Could you check a few things on this model? Use its own coordinates, in mm. Face numbers are marked on the shaded views. A direction names the side the tool comes from. Give positions to 0.01 mm unless a question says otherwise; leave off trailing zeros. Loops run counter-clockwise (first coordinate to the right, second up) from the corner with the lowest first, then second, coordinate; pieces in that order, holes last. Notation, with made-up numbers: M 63.25,17 L 113.25,17 A22 ccw 113.25,47 Z; hole C 77.25,5.25 d1. An arc over 180 degrees is marked long. Return JSON: item names as keys, results as strings. Group by question number.
1. Please list where these lines run through material, in increasing order: line 1 (X direction, y = 3, z = 32); line 2 (Z direction, x = 47, y = 16); line 3 (X direction, y = 8, z = 11.5).
2. If we mould it in two halves opening along Y, with no side actions, what happens to the marked faces 4, 5, 6 and 7? For each: +Y half, -Y half, draft (parallel to the pull), parting line (faces both ways), or undercut.
3. For the marked faces 1, 2 and 3, which set-ups out of +Z, -Z, +X, -X, +Y, -Y let a thin tool reach every point of the face, with its end or its side?
4. If we section it at B-B (x = 52.5): Write out the boundary of the cut face in (y, z), plus the area to 3 significant figures.
5. If we section it at D-D (z = 40): Write out the boundary of the cut face in (x, y), plus the area to 3 significant figures.
6. If we section it at A-A (z = 11): Write out the boundary of the cut face in (x, y).
7. If we section it at C-C (y = 29.5): Write out the boundary of the cut face in (x, z), plus the area to 3 significant figures.
8. For pin 1 (10 mm diameter, centred on y = 24.5, z = 22.5, fed in from -X); pin 2 (15.5 mm diameter, centred on y = 16.5, z = 14, fed in from -X); pin 3 (0.7 mm diameter, centred on x = 30, z = 7.5, fed in from -Y), each with a flat end and sliding along its axis, tell me the tip position at first contact or that it passes through.
```python
from build123d import *

# Parameters (mm, degrees)
F0_W      = 58
F0_H      = 33
F1_DEPTH  = 2
F2_R      = 10
F3_DEPTH  = 15
F4_R      = 4.7
F5_DEPTH  = 14
F6_W      = 12
F6_H      = 1.5
F7_DEPTH  = 34.5
F8_W      = 1.2
F8_H      = 33
F9_DEPTH  = 45
F10_R     = 4.75
F11_DEPTH = 20
F12_W     = 1.2
F12_H     = 33
F13_DEPTH = 45
F14_R     = 9.6
F15_DEPTH = 10
F17_DEPTH = 1.2
F19_DEPTH = 1.2
F20_W     = 9
F20_H     = 45
F21_DEPTH = 1.2
F22_W     = 9
F22_H     = 45
F23_DEPTH = 1.2
F24_SIZE  = 5


with BuildPart() as f1:
    # F0 (on Top) → F1 (new body)
    with BuildSketch(Plane.XY):
        with Locations((29, 16.5)):
            Rectangle(F0_W, F0_H)
    extrude(amount=F1_DEPTH)

    # F2 (on face) → F3 (join)
    with BuildSketch(Plane.XY.offset(2)):
        with Locations((29, 16.5)):
            Circle(F2_R)
    extrude(amount=F3_DEPTH)

    # F4 (on face) → F5 (cut)
    with BuildSketch(Plane.XY.offset(17)):
        with Locations((29, 16.5)):
            Circle(F4_R)
    extrude(amount=-F5_DEPTH, mode=Mode.SUBTRACT)

    # F6 (on Right) → F7 (cut)
    with BuildSketch(Plane.YZ):
        with Locations((15.833333, 7.95)):
            Rectangle(F6_W, F6_H)
    extrude(amount=F7_DEPTH, mode=Mode.SUBTRACT)

    # F8 (on face) → F9 (join)
    with BuildSketch(Plane.XY.offset(2)):
        with Locations((57.4, 16.5)):
            Rectangle(F8_W, F8_H)
    extrude(amount=F9_DEPTH)

    # F10 (on face) → F11 (cut)
    with BuildSketch(Plane.YZ.offset(58)):
        with Locations((16.5, 27)):
            Circle(F10_R)
    extrude(amount=-F11_DEPTH, mode=Mode.SUBTRACT)

    # F12 (on face) → F13 (join)
    with BuildSketch(Plane.XY.offset(2)):
        with Locations((47.2, 16.5)):
            Rectangle(F12_W, F12_H)
    extrude(amount=F13_DEPTH)

    # F14 (on face) → F15 (cut)
    with BuildSketch(Plane.YZ.offset(47.8)):
        with Locations((16.5, 27)):
            Circle(F14_R)
    extrude(amount=-F15_DEPTH, mode=Mode.SUBTRACT)

    # F16 (on Front) → F17 (join)
    with BuildSketch(Plane.XZ):
        Polygon((46.6, 2), (46.6, 47), (29.1, 2), align=None)
    extrude(amount=-F17_DEPTH)

    # F18 (on face) → F19 (join)
    with BuildSketch(Plane(origin=(0, 33, 0), x_dir=(-1, 0, 0), z_dir=(0, 1, 0))):
        Polygon((-29, 2), (-46.6, 47), (-46.6, 2), align=None)
    extrude(amount=-F19_DEPTH)

    # F20 (on Front) → F21 (join)
    with BuildSketch(Plane.XZ):
        with Locations((52.3, 24.5)):
            Rectangle(F20_W, F20_H)
    extrude(amount=-F21_DEPTH)

    # F22 (on face) → F23 (join)
    with BuildSketch(Plane(origin=(0, 33, 0), x_dir=(-1, 0, 0), z_dir=(0, 1, 0))):
        with Locations((-52.3, 24.5)):
            Rectangle(F22_W, F22_H)
    extrude(amount=-F23_DEPTH)

    # F24
    f24_edges = [f1.edges().sort_by_distance(p)[0] for p in [
        (19, 16.5, 17),
    ]]
    chamfer(f24_edges, length=F24_SIZE)


solid = f1.part
```
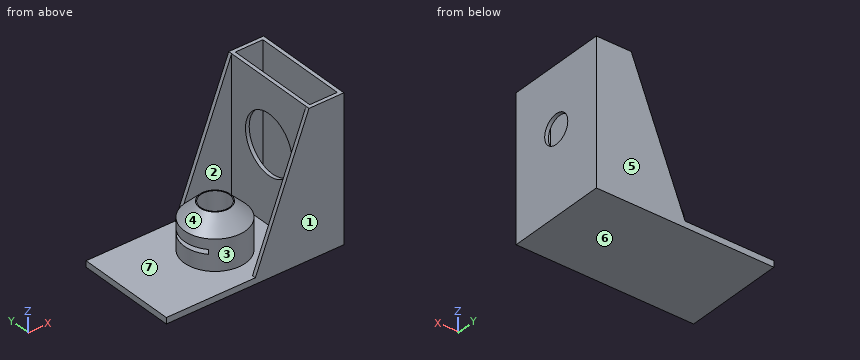
Answer:
{
 "1": {"line 1": "x = 46.6 to 47.8, 56.8 to 58", "line 2": "z = 0 to 17.41, 36.59 to 47", "line 3": "x = 23.73 to 34.27, 46.6 to 47.8, 56.8 to 58"},
 "2": {"face 4": "undercut", "face 5": "+Y half", "face 6": "draft", "face 7": "undercut"},
 "3": {"face 1": "+Z, -Z, +X, -X, -Y", "face 2": "+Z, -X", "face 3": "+Z"},
 "4": {"outline": "M 0,0 L 33,0 L 33,47 L 31.8,47 L 31.8,2 L 1.2,2 L 1.2,47 L 0,47 Z", "area": "174 mm²"},
 "5": {"outline": "M 43.86,31.8 L 46.6,31.8 L 46.6,1.2 L 43.88,1.2 L 43.88,0 L 58,0 L 58,33 L 43.86,33 Z; hole M 47.8,1.2 L 56.8,1.2 L 56.8,31.8 L 47.8,31.8 Z", "area": "107 mm²"},
 "6": {"outline": "C 29,16.5 d20; M 32.52,31.8 L 46.6,31.8 L 46.6,1.2 L 32.6,1.2 L 32.6,0 L 58,0 L 58,33 L 32.52,33 Z; hole C 29,16.5 d9.4; hole M 47.8,1.2 L 56.8,1.2 L 56.8,31.8 L 47.8,31.8 Z"},
 "7": {"outline": "M 0,0 L 58,0 L 58,47 L 56.8,47 L 56.8,2 L 47.8,2 L 47.8,47 L 46.6,47 L 46.6,2 L 0,2 Z", "area": "224 mm²"},
 "8": {"pin 1": "stops at x = 46.6", "pin 2": "stops at x = 19", "pin 3": "stops at y = 6.52"}
}
